Input: part model. Units: mm. Frame: model coordinates. A direction names the side the tool comes from. Give positions to 0.01 mm unless a question says otherwise; leave off trailing zeros. Order: outer loops, then holes, each group sorted by start corner. A loop starts at its lowest first (then second) coordinate and runs counter-clockwise, first axis right, second up. Notation, with made-up numbers: (46, 23) - (51, 23) arc R25 ccw to (51, 61) - close; hole circle Ø10 at (36, -36). An arc over 180 degrees is marked (long way). Answer in a Markdown table with one row per item. Add a question column.
1. Section query A-A on x = -3. Return loops of the section in (y, z), and give its area (3 significant figures).
2. Mould query, pull axis Y, two halves, no side actions, for faces 1 (the face through (125, -38, 42.862)), 2 (the face through (95, -48, 42.862)). Classes: released by +Y, released by -Y, zero draft, split by the parting line, or undercut.
3. Access query for faces 3 (the face through (-57, 48, 42.862)), 4 (the face through (-125, 19, 42.862)), 5 (the face through (-12.7, -48, 24)), 6 (the face through (-95.25, 0, 30)). Directions: +Z, -Z, +X, -X, +Y, -Y. A direction counts if a zero-diameter tool reaches every point of the face in a straight line with its end or side. Return the directions, or none.
4. Ray query, line 1 (Y direction, x = -82, z = 53.5); line 2 (X direction, y = 1, z = 50); line 3 (Y direction, x = -57, z = 17). Return the intervals inside material, ascending. Write a range as [from, to].
5. Section query D-D on y = 28. Return loops of the section in (x, z).
6. Section query C-C on z = 28. Count the separate pieces of the cut face and the enclosed holes in it, and give its area (3 significant figures).
7. Section query B-B on x = -112. Return loops of the section in (y, z), and give its area (3 significant figures).
8. Contact query for flat-ended pins moving along their axis: pin 1 (2.5 mm diameter, centred on y = 49.5, z = 16, fed in from +X); pin 2 (15 mm diameter, centred on x = -1, z = 30.5, fed in from +Y); pin 3 (1.4 mm diameter, centred on x = 123.5, z = 26, fed in from -Y); pin 4 (2.5 mm diameter, centred on x = 41, y = 48, fed in from -Z). Output: stop coordinate, or through.
```python
from build123d import *

# Parameters (mm, degrees)
F0_W     = 266.7
F0_H     = 114.3
F1_DEPTH = 4.7625
F2_W     = 4.7625
F2_H     = 6.35
F2_W_2   = 6.35
F2_H_2   = 4.7625
F3_DEPTH = 38.1
F5_DEPTH = 12.7
F6_W     = 4.7625
F6_H     = 6.35
F6_W_2   = 6.35
F6_H_2   = 4.7625
F6_W_3   = 190.5
F6_H_3   = 38.1
F6_W_4   = 180.975
F6_H_4   = 28.575
F7_DEPTH = 50.8
F9_DEPTH = 266.7


with BuildPart() as f1:
    # F0 (on Top) → F1 (new body)
    with BuildSketch(Plane.XY):
        Rectangle(F0_W, F0_H)
    extrude(amount=F1_DEPTH)

    # F2 (on face) → F3 (join)
    with BuildSketch(Plane.XY.offset(4.7625)):
        with Locations((124.61875, -47.625)):
            Rectangle(F2_W, F2_H)
        with Locations((124.61875, 9.525)):
            Rectangle(F2_W, F2_H)
        with Locations((124.61875, 28.575)):
            Rectangle(F2_W, F2_H)
        with Locations((124.61875, -9.525)):
            Rectangle(F2_W, F2_H)
        with Locations((124.61875, -28.575)):
            Rectangle(F2_W, F2_H)
        with Locations((-124.61875, 47.625)):
            Rectangle(F2_W, F2_H)
        with Locations((-104.775, 48.41875)):
            Rectangle(F2_W_2, F2_H_2)
        with Locations((-85.725, 48.41875)):
            Rectangle(F2_W_2, F2_H_2)
        with Locations((-66.675, 48.41875)):
            Rectangle(F2_W_2, F2_H_2)
        with Locations((-47.625, 48.41875)):
            Rectangle(F2_W_2, F2_H_2)
        with Locations((-28.575, 48.41875)):
            Rectangle(F2_W_2, F2_H_2)
        with Locations((9.525, 48.41875)):
            Rectangle(F2_W_2, F2_H_2)
        with Locations((28.575, 48.41875)):
            Rectangle(F2_W_2, F2_H_2)
        with Locations((47.625, 48.41875)):
            Rectangle(F2_W_2, F2_H_2)
        with Locations((66.675, 48.41875)):
            Rectangle(F2_W_2, F2_H_2)
        with Locations((85.725, 48.41875)):
            Rectangle(F2_W_2, F2_H_2)
        with Locations((104.775, 48.41875)):
            Rectangle(F2_W_2, F2_H_2)
        with Locations((124.61875, 47.625)):
            Rectangle(F2_W, F2_H)
        with Locations((-9.525, 48.41875)):
            Rectangle(F2_W_2, F2_H_2)
        with Locations((-124.61875, 28.575)):
            Rectangle(F2_W, F2_H)
        with Locations((-124.61875, 9.525)):
            Rectangle(F2_W, F2_H)
        with Locations((-124.61875, -9.525)):
            Rectangle(F2_W, F2_H)
        with Locations((-124.61875, -47.625)):
            Rectangle(F2_W, F2_H)
        with Locations((-104.775, -48.41875)):
            Rectangle(F2_W_2, F2_H_2)
        with Locations((-85.725, -48.41875)):
            Rectangle(F2_W_2, F2_H_2)
        with Locations((-124.61875, -28.575)):
            Rectangle(F2_W, F2_H)
        with Locations((-66.675, -48.41875)):
            Rectangle(F2_W_2, F2_H_2)
        with Locations((-47.625, -48.41875)):
            Rectangle(F2_W_2, F2_H_2)
        with Locations((-28.575, -48.41875)):
            Rectangle(F2_W_2, F2_H_2)
        with Locations((-9.525, -48.41875)):
            Rectangle(F2_W_2, F2_H_2)
        with Locations((9.525, -48.41875)):
            Rectangle(F2_W_2, F2_H_2)
        with Locations((28.575, -48.41875)):
            Rectangle(F2_W_2, F2_H_2)
        with Locations((47.625, -48.41875)):
            Rectangle(F2_W_2, F2_H_2)
        with Locations((66.675, -48.41875)):
            Rectangle(F2_W_2, F2_H_2)
        with Locations((85.725, -48.41875)):
            Rectangle(F2_W_2, F2_H_2)
        with Locations((104.775, -48.41875)):
            Rectangle(F2_W_2, F2_H_2)
    extrude(amount=F3_DEPTH)

    # F4 (on face) → F5 (join)
    with BuildSketch(Plane.XY.offset(42.8625)):
        Polygon((127, -50.8), (127, 50.8), (122.2375, 50.8), (122.2375, 46.0375), (122.2375, 44.45), (122.2375, -46.0375), (-122.2375, -46.0375), (-122.2375, -50.8), align=None)
        Polygon((122.2375, 46.0375), (122.2375, 50.8), (-127, 50.8), (-127, -50.8), (-122.2375, -50.8), (-122.2375, -46.0375), (-122.2375, -44.45), (-122.2375, 46.0375), align=None)
    extrude(amount=F5_DEPTH)

    # F6 (on face) → F7 (join)
    with BuildSketch(Plane.XY.offset(4.7625)):
        with Locations((124.61875, 28.575)):
            Rectangle(F6_W, F6_H)
        with Locations((124.61875, 9.525)):
            Rectangle(F6_W, F6_H)
        with Locations((124.61875, -9.525)):
            Rectangle(F6_W, F6_H)
        with Locations((124.61875, -28.575)):
            Rectangle(F6_W, F6_H)
        with Locations((124.61875, 47.625)):
            Rectangle(F6_W, F6_H)
        with Locations((124.61875, -47.625)):
            Rectangle(F6_W, F6_H)
        with Locations((-124.61875, -47.625)):
            Rectangle(F6_W, F6_H)
        with Locations((9.525, -48.41875)):
            Rectangle(F6_W_2, F6_H_2)
        with Locations((-66.675, -48.41875)):
            Rectangle(F6_W_2, F6_H_2)
        with Locations((47.625, -48.41875)):
            Rectangle(F6_W_2, F6_H_2)
        with Locations((-28.575, -48.41875)):
            Rectangle(F6_W_2, F6_H_2)
        with Locations((-104.775, -48.41875)):
            Rectangle(F6_W_2, F6_H_2)
        with Locations((-85.725, -48.41875)):
            Rectangle(F6_W_2, F6_H_2)
        with Locations((-9.525, -48.41875)):
            Rectangle(F6_W_2, F6_H_2)
        with Locations((66.675, -48.41875)):
            Rectangle(F6_W_2, F6_H_2)
        with Locations((85.725, -48.41875)):
            Rectangle(F6_W_2, F6_H_2)
        with Locations((104.775, -48.41875)):
            Rectangle(F6_W_2, F6_H_2)
        with Locations((-47.625, -48.41875)):
            Rectangle(F6_W_2, F6_H_2)
        with Locations((28.575, -48.41875)):
            Rectangle(F6_W_2, F6_H_2)
        with Locations((-124.61875, 28.575)):
            Rectangle(F6_W, F6_H)
        with Locations((-124.61875, 9.525)):
            Rectangle(F6_W, F6_H)
        with Locations((-124.61875, -9.525)):
            Rectangle(F6_W, F6_H)
        with Locations((-124.61875, -28.575)):
            Rectangle(F6_W, F6_H)
        with Locations((-124.61875, 47.625)):
            Rectangle(F6_W, F6_H)
        with Locations((104.775, 48.41875)):
            Rectangle(F6_W_2, F6_H_2)
        with Locations((47.625, 48.41875)):
            Rectangle(F6_W_2, F6_H_2)
        with Locations((85.725, 48.41875)):
            Rectangle(F6_W_2, F6_H_2)
        with Locations((66.675, 48.41875)):
            Rectangle(F6_W_2, F6_H_2)
        with Locations((28.575, 48.41875)):
            Rectangle(F6_W_2, F6_H_2)
        with Locations((9.525, 48.41875)):
            Rectangle(F6_W_2, F6_H_2)
        with Locations((-9.525, 48.41875)):
            Rectangle(F6_W_2, F6_H_2)
        with Locations((-28.575, 48.41875)):
            Rectangle(F6_W_2, F6_H_2)
        with Locations((-47.625, 48.41875)):
            Rectangle(F6_W_2, F6_H_2)
        with Locations((-66.675, 48.41875)):
            Rectangle(F6_W_2, F6_H_2)
        with Locations((-85.725, 48.41875)):
            Rectangle(F6_W_2, F6_H_2)
        with Locations((-104.775, 48.41875)):
            Rectangle(F6_W_2, F6_H_2)
        Rectangle(F6_W_3, F6_H_3)
        Rectangle(F6_W_4, F6_H_4, mode=Mode.SUBTRACT)
    extrude(amount=F7_DEPTH)

    # F8 (on face) → F9 (join, through all)
    with BuildSketch(Plane.YZ.offset(133.35)):
        Polygon((-57.15, 55.5625), (-50.8, 55.5625), (50.8, 55.5625), (57.15, 55.5625), (57.15, 58.7375), (0, 74.6125), (-57.15, 58.7375), align=None)
    extrude(amount=-F9_DEPTH)


solid = f1.part
```
Answer:
| question | item | result |
|---|---|---|
| 1 | outline | (-57.15, 0) - (57.15, 0) - (57.15, 4.76) - (19.05, 4.76) - (19.05, 55.56) - (46.04, 55.56) - (46.04, 42.86) - (50.8, 42.86) - (50.8, 55.56) - (57.15, 55.56) - (57.15, 58.74) - (0, 74.61) - (-57.15, 58.74) - (-57.15, 55.56) - (-50.8, 55.56) - (-50.8, 42.86) - (-46.04, 42.86) - (-46.04, 55.56) - (-19.05, 55.56) - (-19.05, 4.76) - (-57.15, 4.76) - close; hole (-14.29, 4.76) - (14.29, 4.76) - (14.29, 55.56) - (-14.29, 55.56) - close |
| 1 | area | 2,420 mm² |
| 2 | face 1 | undercut |
| 2 | face 2 | zero draft |
| 3 | face 3 | +Y |
| 3 | face 4 | -X |
| 3 | face 5 | -Y |
| 3 | face 6 | none |
| 4 | line 1 | y = [-50.8, -46.04], [-19.05, -14.29], [14.29, 19.05], [46.04, 50.8] |
| 4 | line 2 | x = [-127, -122.24], [-95.25, -90.49], [90.49, 95.25], [122.24, 127] |
| 4 | line 3 | y = [-19.05, -14.29], [14.29, 19.05] |
| 5 | outline | (-133.35, 0) - (133.35, 0) - (133.35, 4.76) - (127, 4.76) - (127, 55.56) - (133.35, 55.56) - (133.35, 66.83) - (-133.35, 66.83) - (-133.35, 55.56) - (-127, 55.56) - (-127, 4.76) - (-133.35, 4.76) - close; hole (-122.24, 4.76) - (122.24, 4.76) - (122.24, 55.56) - (-122.24, 55.56) - close |
| 6 | separate pieces | 37 |
| 6 | enclosed holes | 1 |
| 6 | area | 3,180 mm² |
| 7 | outline | (-57.15, 0) - (57.15, 0) - (57.15, 4.76) - (-57.15, 4.76) - close; (-57.15, 55.56) - (-50.8, 55.56) - (-50.8, 42.86) - (-46.04, 42.86) - (-46.04, 55.56) - (46.04, 55.56) - (46.04, 42.86) - (50.8, 42.86) - (50.8, 55.56) - (57.15, 55.56) - (57.15, 58.74) - (0, 74.61) - (-57.15, 58.74) - close |
| 7 | area | 1,940 mm² |
| 8 | pin 1 | stops at x = 127 |
| 8 | pin 2 | stops at y = 50.8 |
| 8 | pin 3 | stops at y = -50.8 |
| 8 | pin 4 | stops at z = 0 |
